```python
from build123d import *

# Parameters (mm, degrees)
SKETCH1_W           = 72
SKETCH1_H           = 57
BOSS_EXTRUDE1_DEPTH = 5
BOSS_EXTRUDE2_DEPTH = 12
SKETCH5_R           = 2.25
CUT_EXTRUDE2_DEPTH  = 64.790673299
SKETCH4_R           = 12
SKETCH4_R_2         = 1.75
CUT_EXTRUDE1_DEPTH  = 64.120915709
SKETCH6_R           = 2.25
CUT_EXTRUDE3_DEPTH  = 64.120915709
SKETCH7_W           = 30
SKETCH7_H           = 10
BOSS_EXTRUDE3_DEPTH = 17
BOSS_EXTRUDE4_START = -5
BOSS_EXTRUDE4_DEPTH = 5
SKETCH9_W           = 10
SKETCH9_H           = 3
CUT_EXTRUDE4_DEPTH  = 66.094162565


with BuildPart() as part:
    # Sketch1 → Boss-Extrude1 (new body)
    with BuildSketch(Plane.XY):
        with Locations((-20, 0)):
            Rectangle(SKETCH1_W, SKETCH1_H)
    extrude(amount=BOSS_EXTRUDE1_DEPTH)

    # Sketch3 → Boss-Extrude2 (add)
    with BuildSketch(Plane(origin=(16, 0, 0), x_dir=(0, 0, -1), z_dir=(1, 0, 0))):
        with BuildLine():
            Line((-5, 28.5), (-11, 28.5))
            Line((-11, 28.5), (-11, 20.5))
            ThreePointArc((-11, 20.5), (-7, 16.5), (-11, 12.5))
            Line((-11, 12.5), (-11, 4.5))
            Line((-11, 4.5), (-5, 4.5))
            Line((-5, 4.5), (-5, 28.5))
        make_face()
    boss_extrude2 = extrude(amount=-BOSS_EXTRUDE2_DEPTH)

    # Sketch5 → Cut-Extrude2 (cut, through all)
    with BuildSketch(Plane.XY.offset(11)):
        with Locations((10, 24.5)):
            Circle(SKETCH5_R)
        with Locations((10, 8.5)):
            Circle(SKETCH5_R)
    cut_extrude2 = extrude(amount=-CUT_EXTRUDE2_DEPTH, mode=Mode.SUBTRACT)

    # Mirror1: Boss-Extrude2, Cut-Extrude2 across plane
    add(boss_extrude2.mirror(Plane(origin=(0, 0, 0), x_dir=(0, 0, 1), z_dir=(1, 0, 0))))
    add(cut_extrude2.mirror(Plane(origin=(0, 0, 0), x_dir=(0, 0, 1), z_dir=(1, 0, 0))), mode=Mode.SUBTRACT)

    # Sketch4 → Cut-Extrude1 (cut, through all)
    with BuildSketch(Plane.XY.offset(5)):
        with Locations((-35, -6.5)):
            Circle(SKETCH4_R)
        with Locations((-50.5, 9)):
            Circle(SKETCH4_R_2)
        with Locations((-19.5, 9)):
            Circle(SKETCH4_R_2)
        with Locations((-19.5, -22)):
            Circle(SKETCH4_R_2)
        with Locations((-50.5, -22)):
            Circle(SKETCH4_R_2)
    extrude(amount=-CUT_EXTRUDE1_DEPTH, mode=Mode.SUBTRACT)

    # Sketch6 → Cut-Extrude3 (cut, through all)
    with BuildSketch(Plane.XY.offset(5)):
        with Locations((-7, -22.5)):
            Circle(SKETCH6_R)
        with Locations((11, -22.5)):
            Circle(SKETCH6_R)
    extrude(amount=-CUT_EXTRUDE3_DEPTH, mode=Mode.SUBTRACT)

    # Sketch7 → Boss-Extrude3 (add)
    with BuildSketch(Plane.XY.offset(5)):
        with Locations((-41, 23.5)):
            Rectangle(SKETCH7_W, SKETCH7_H)
    extrude(amount=BOSS_EXTRUDE3_DEPTH)

    # Sketch8 → Boss-Extrude4 (add)
    with BuildSketch(Plane(origin=(-26, 0, 0), x_dir=(0, 0, -1), z_dir=(1, 0, 0)).offset(BOSS_EXTRUDE4_START)):
        Polygon((-22, 18.5), (-5, 8.5), (-5, 18.5), align=None)
    extrude(amount=-BOSS_EXTRUDE4_DEPTH)

    # Sketch9 → Cut-Extrude4 (cut, through all)
    with BuildSketch(Plane.XY.offset(5)):
        with Locations((-41, 17)):
            Rectangle(SKETCH9_W, SKETCH9_H)
    extrude(amount=-CUT_EXTRUDE4_DEPTH, mode=Mode.SUBTRACT)


solid = part.part
```
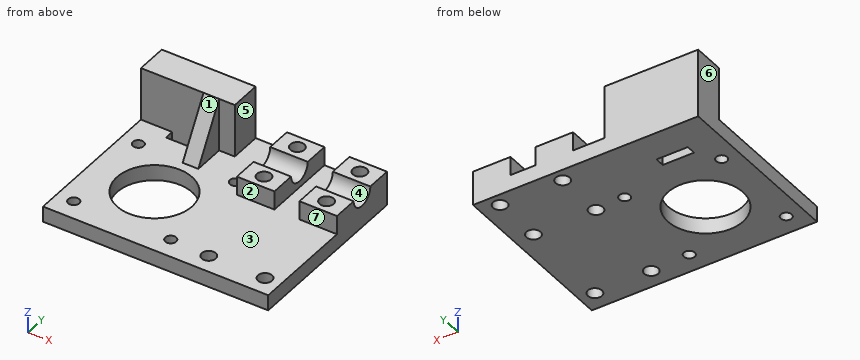
Can you work these out from the model? Positions are in its coordinate system, mm. Face numbers are marked on the shaded views. A direction names the side the tool comes from. Round coordinates to 2 decimals unless told otherwise and drop trailing zeros. Loops run counter-clockwise (first coordinate to the right, second up) from the corner with the lowest first, then second, coordinate; pieces in that order, holes last. Notation, with made-up numbers: M -23.5,54 L -17.5,54 A29 ccw -17.5,87 Z; hole C 12,53.25 d7. An arc over 180 degrees is marked long. Answer as a JSON object with one key per item and string values. Group by question number.
Q1. Imagine slicing it at D-D, the plane x = -32.5. Please give me the cut outline in (y, z).
Q2. On a 3-axis mill with a long thin cutter (end or side, diameter ignored), from which of +Z, -Z, +X, -X, +Y, -Y can I reach the whole of each face in a straight line? I mean the marked faces 1, 2, 3 and 4. Say none if no direction works.
Q3. Will these pins go through, and if not, where does the flat tip stop? pin 1 (5 mm diameter, centred on y = 15, z = 15, fed in from +X); pin 2 (3 mm diameter, centred on y = -6, z = 6, fed in from -X); pin 3 (2.5 mm diameter, centred on x = -29, z = 15.5, fed in from -Y); pin 4 (3.5 mm diameter, centred on x = 10, y = 8.5, fed in from -Z).
Q4. We'd pull the mould along X, two halves only. Please class the marked faces 5, 6 and 7: +X half, -X half, draft (parallel to the pull), parting line (faces both ways), or undercut.
Q5. Imagine slicing it at A-A, the plane y = 16.5. Please give me the cut outline in (x, z).
Q6. Imagine slicing it at B-B, the plane x = -19.5. Please give me the cut outline in (y, z).
Q7. Please list where these lines run through material, in increasing order: L1, parallel to Y at x = -10, z = 5.5; L2, parallel to Y at x = -50.5, z = 2.8; L3, parallel to Y at x = 9, z = 9.5.
Q8. Imagine slicing it at C-C, the plane z = 1.5. Count the separate pieces of the cut face and the enclosed holes in it, then the cut area to 3 significant figures.
Findings:
{
 "1": {"outline": "M -28.5,0 L -18.24,0 L -18.24,5 L -28.5,5 Z; M 5.24,0 L 28.5,0 L 28.5,22 L 18.5,22 L 8.5,5 L 5.24,5 Z"},
 "2": {"face 1": "+Z, -X, -Y", "face 2": "+Z, +X, -X, -Y", "face 3": "+Z, -Y", "face 4": "+Z, +X"},
 "3": {"pin 1": "stops at x = -31", "pin 2": "stops at x = -56", "pin 3": "stops at y = 18.5", "pin 4": "passes through"},
 "4": {"face 5": "undercut", "face 6": "-X half", "face 7": "draft"},
 "5": {"outline": "M -56,0 L -46,0 L -46,5 L -56,5 Z; M -36,0 L 16,0 L 16,7 L 4,7 L 4,5 L -4,5 L -4,7 L -16,7 L -16,5 L -31,5 L -31,18.6 L -36,18.6 Z"},
 "6": {"outline": "M -28.5,0 L -23.75,0 L -23.75,5 L -28.5,5 Z; M -20.25,0 L 7.25,0 L 7.25,5 L -20.25,5 Z; M 10.75,0 L 28.5,0 L 28.5,5 L 10.75,5 Z"},
 "7": {"L1": "y = 4.5 to 6.25, 10.75 to 22.25, 26.75 to 28.5", "L2": "y = -28.5 to -23.75, -20.25 to 7.25, 10.75 to 28.5", "L3": "y = 4.5 to 6.48, 10.52 to 12.79, 20.21 to 22.48, 26.52 to 28.5"},
 "8": {"separate pieces": "1", "enclosed holes": "12", "area": "3,490 mm2"}
}
